```python
from build123d import *

# Parameters (mm, degrees)
F0_W     = 80
F0_H     = 48
F1_DEPTH = 20
F2_R     = 7.5
F3_DEPTH = 20.001
F4_W     = 19.5
F4_H     = 23
F5_DEPTH = 20.001
F6_R     = 5.5
F6_R_2   = 4
F7_DEPTH = 6
F8_DEPTH = 25.001


with BuildPart() as f1:
    # F0 (on Right) → F1 (new body)
    with BuildSketch(Plane.YZ):
        Rectangle(F0_W, F0_H)
    extrude(amount=F1_DEPTH)

    # F2 (on face) → F3 (cut, through all)
    with BuildSketch(Plane.YZ.offset(20)):
        with Locations((0, 4)):
            Circle(F2_R)
    extrude(amount=-F3_DEPTH, mode=Mode.SUBTRACT)

    # F4 (on face) → F5 (cut, through all)
    with BuildSketch(Plane.YZ.offset(20)):
        with Locations((-30.25, 12.5)):
            Rectangle(F4_W, F4_H)
        with Locations((30.25, 12.5)):
            Rectangle(F4_W, F4_H)
    extrude(amount=-F5_DEPTH, mode=Mode.SUBTRACT)

    # F6 (on face) → F7 (cut)
    with BuildSketch(Plane.XY.offset(1)):
        with Locations((10, 30)):
            Circle(F6_R)
        with Locations((10, 30)):
            Circle(F6_R_2, mode=Mode.SUBTRACT)
        with Locations((10, -30)):
            Circle(F6_R)
        with Locations((10, -30)):
            Circle(F6_R_2, mode=Mode.SUBTRACT)
    extrude(amount=-F7_DEPTH, mode=Mode.SUBTRACT)

    # F8 (cut, through all): faces of the model
    f8_faces = [f1.faces().sort_by_distance(p)[0] for p in [
        (10, 30, 1),
        (10, -30, 1),
    ]]
    extrude(f8_faces, amount=-F8_DEPTH, mode=Mode.SUBTRACT)


solid = f1.part
```
Could you check a few things on this model? Use its own coordinates, in mm. A direction names the side the tool comes from. Round coordinates to 2 decimals unless told otherwise and drop trailing zeros. Loops run counter-clockwise (first coordinate to the right, second up) from the corner with the lowest first, then second, coordinate; pieces in that order, holes last. Notation, with made-up numbers: (-33.5, -7.75) - (15.5, -7.75) arc R16 ccw to (15.5, 18.25) - close; hole circle Ø9 at (22.25, 26.25). An arc over 180 degrees is marked (long way). Answer in a Markdown table with one row per item. Add a question column.
(1) For faces 5 (the face through (15, 26, 1)), 6 (the face through (15.246, -28.348, -1.958)), 7 (the face through (15, -35, 1)), which set-ups out of +Z, -Z, +X, -X, +Y, -Y let a thin tool reach every point of the face, with its end or its side?
(2) If we section it at C-C (z = 4): Please give me the cut outline in (x, y), plus the area to 3 significant figures.
(3) If we section it at D-D (z = -12): Please give me the cut outline in (x, y), plus the area to 3 significant figures.
(4) If we section it at A-A (x = 10): Please give me the cut outline in (y, z), plus the area to 3 significant figures.
(5) I'm going to push flat-ended pins straight in: pin 1 (4 mm diameter, centred on y = -23, z = -18, fed in from -X); pin 2 (9 mm diameter, centred on x = 7.5, y = -30, fed in from +Z). Where does each tip first touch, or does it pass through?
(6) I need wall thicknesses on line 1 along Y through (x, z) = (10, -19.5); line 2 along Y through (x, z) = (10, -0.85); line 3 along Z through (x, y) = (15.5, 0). Which ranges of each line are inside material? Lowest first, please.
(7) If we mould it in two halves opening along Y, with no side actions, what happens to faces 1 (the face through (10, -40, -12)), 2 (the face through (9.479, 33.966, -14.367)), 3 (the face through (10, 40, -12)), 4 (the face through (6, -32, -5))? For each: pulls with the +Y half, pulls with the -Y half, needs draft (parallel to the pull), parting line crosses it, or undercut.
(8) If we section it at B-B (y = 0): Please give me the cut outline in (x, z), plus the area to 3 significant figures.
Model answer:
| question | item | result |
|---|---|---|
| 1 | face 5 | +Z, +X, -X, +Y |
| 1 | face 6 | +Z |
| 1 | face 7 | +Z, +X, -X, -Y |
| 2 | outline | (0, -20.5) - (20, -20.5) - (20, -7.5) - (0, -7.5) - close; (0, 7.5) - (20, 7.5) - (20, 20.5) - (0, 20.5) - close |
| 2 | area | 520 mm² |
| 3 | outline | (0, -40) - (20, -40) - (20, 40) - (0, 40) - close; hole circle Ø8 at (10, -30); hole circle Ø8 at (10, 30) |
| 3 | area | 1,500 mm² |
| 4 | outline | (-40, -24) - (-34, -24) - (-34, -5) - (-35.5, -5) - (-35.5, 1) - (-40, 1) - close; (-26, -24) - (26, -24) - (26, -5) - (24.5, -5) - (24.5, 1) - (20.5, 1) - (20.5, 24) - (-20.5, 24) - (-20.5, 1) - (-24.5, 1) - (-24.5, -5) - (-26, -5) - close; (34, -24) - (40, -24) - (40, 1) - (35.5, 1) - (35.5, -5) - (34, -5) - close; hole circle Ø15 at (0, 4) |
| 4 | area | 2,330 mm² |
| 5 | pin 1 | stops at x = 0 |
| 5 | pin 2 | stops at z = 1 |
| 6 | line 1 | y = -40 to -34, -26 to 26, 34 to 40 |
| 6 | line 2 | y = -40 to -35.5, -24.5 to -5.72, 5.72 to 24.5, 35.5 to 40 |
| 6 | line 3 | z = -24 to -3.5, 11.5 to 24 |
| 7 | face 1 | pulls with the -Y half |
| 7 | face 2 | undercut |
| 7 | face 3 | pulls with the +Y half |
| 7 | face 4 | undercut |
| 8 | outline | (0, -24) - (20, -24) - (20, -3.5) - (0, -3.5) - close; (0, 11.5) - (20, 11.5) - (20, 24) - (0, 24) - close |
| 8 | area | 660 mm² |
